Geometry: final body of the model. Coordinates: model frame, mm. A direction names the side the tool comes from. Coordinates: 2 decimals unless noted, no trailing zeros. Loops run counter-clockwise (first coordinate to the right, second up) from the corner with the lowest first, then second, coordinate; pieces in that order, holes last. Notation, with made-up numbers: (7, 15) - (14, 15) arc R25 cw to (14, 31) - close; hole circle Ø4 at (8, 62). An arc over 180 degrees is marked (long way). Answer in a Markdown table with one row per item.
from build123d import *

# Parameters (mm, degrees)
BOSS_EXTRUDE1_DEPTH   = 25.4
F_6_32_TAPPED_HOLE1_D = 2.7051
F_6_32_TAPPED_HOLE2_D = 2.7051
SKETCH7_R             = 1.5875
CUT_EXTRUDE1_DEPTH    = 4.048


with BuildPart() as part:
    # Sketch1 → Boss-Extrude1 (new body)
    with BuildSketch(Plane.XY):
        Polygon((0, 0), (19.05, 0), (19.05, 3.048), (3.048, 3.048), (3.048, 19.05), (0, 19.05), align=None)
    extrude(amount=BOSS_EXTRUDE1_DEPTH)

    # #6-32 Tapped Hole1 (through all)
    with Locations(Plane(origin=(3.048, 0, 0), x_dir=(0, 0, -1), z_dir=(1, 0, 0))):
        with Locations((-20.32, 9.525), (-5.08, 9.525)):
            Hole(F_6_32_TAPPED_HOLE1_D / 2)

    # #6-32 Tapped Hole2 (through all)
    with Locations(Plane(origin=(0, 3.048, 0), x_dir=(1, 0, 0), z_dir=(0, 1, 0))):
        with Locations((6, -20.65), (6, -4.65)):
            Hole(F_6_32_TAPPED_HOLE2_D / 2)

    # Sketch7 → Cut-Extrude1 (cut, through all)
    with BuildSketch(Plane(origin=(3.048, 0, 0), x_dir=(0, 0, -1), z_dir=(1, 0, 0))):
        with Locations((-20.32, 14.605)):
            Circle(SKETCH7_R)
        with Locations((-5.08, 14.605)):
            Circle(SKETCH7_R)
    extrude(amount=-CUT_EXTRUDE1_DEPTH, mode=Mode.SUBTRACT)


solid = part.part
(1) Cut plane C-C on z = 4.65. Output: boundary loops of the cut face in (x, y), then the cut area to 3 significant figures.
Verdict:
| item | result |
|---|---|
| outline | (0, 0) - (4.65, 0) - (4.65, 3.05) - (3.05, 3.05) - (3.05, 8.24) - (0, 8.24) - close; (0, 10.81) - (3.05, 10.81) - (3.05, 13.08) - (0, 13.08) - close; (0, 16.13) - (3.05, 16.13) - (3.05, 19.05) - (0, 19.05) - close; (7.35, 0) - (19.05, 0) - (19.05, 3.05) - (7.35, 3.05) - close |
| area | 81.5 mm² |
(2) First-contact query: pin 1 Ø8 at (y, z) = (10.5, 6.5) entering from +X; pin 2 Ø1.9 at (y, z) = (14.605, 5.08) entering from +X; pin 3 Ø5 at (x, z) = (7.5, 5.5) entering from +Y; pin 4 Ø8 at (y, z) = (3.5, 16.5) entering from +X. Flat tips, straight axial feed; report the tip coordinate or a pass-through.
Verdict:
| item | result |
|---|---|
| pin 1 | stops at x = 3.05 |
| pin 2 | passes through |
| pin 3 | stops at y = 3.05 |
| pin 4 | stops at x = 19.05 |
(3) Pull-direction query (X, two-part tool) for faces 3 (the face through (3.048, 11, 13)), 4 (the face through (5.38, 1.5, 21.85)), 5 (the face through (9, 0, 13)); classes: pulls with the +X half, pulls with the -X half, needs draft (parallel to the pull), parting line crosses it, or undercut.
Verdict:
| item | result |
|---|---|
| face 3 | pulls with the +X half |
| face 4 | undercut |
| face 5 | needs draft |
(4) Cut plane B-B on y = 8.5. Output: boundary loops of the cut face in (x, z).
Verdict:
| item | result |
|---|---|
| outline | (0, 0) - (3.05, 0) - (3.05, 4.2) - (0, 4.2) - close; (0, 5.96) - (3.05, 5.96) - (3.05, 19.44) - (0, 19.44) - close; (0, 21.2) - (3.05, 21.2) - (3.05, 25.4) - (0, 25.4) - close |
(5) Cut plane A-A on x = 6. Output: boundary loops of the cut face in (y, z), then the cut area to 3 significant figures.
Verdict:
| item | result |
|---|---|
| outline | (0, 0) - (3.05, 0) - (3.05, 3.3) - (0, 3.3) - close; (0, 6) - (3.05, 6) - (3.05, 19.3) - (0, 19.3) - close; (0, 22) - (3.05, 22) - (3.05, 25.4) - (0, 25.4) - close |
| area | 60.9 mm² |
(6) Cut plane D-D on z = 14. Output: boundary loops of the cut face in (x, y), then the cut area to 3 significant figures.
Verdict:
| item | result |
|---|---|
| outline | (0, 0) - (19.05, 0) - (19.05, 3.05) - (3.05, 3.05) - (3.05, 19.05) - (0, 19.05) - close |
| area | 107 mm² |
(7) Ray query, probe 1 along Z at (x, y) = (6, 1.25); probe 2 along Y at (x, z) = (0.75, 20.32); probe 3 along Z at (x, y) = (3, 16). Return the intervals inside material, ascending.
Verdict:
| item | result |
|---|---|
| probe 1 | z = 0 to 3.3, 6 to 19.3, 22 to 25.4 |
| probe 2 | y = 0 to 8.17, 10.88 to 13.02, 16.19 to 19.05 |
| probe 3 | z = 0 to 4.32, 5.84 to 19.56, 21.08 to 25.4 |
(8) Access query for faces 1 (the face through (11, 3.048, 13)), 2 (the face through (2, 6, 25.4)). Directions: +Z, -Z, +X, -X, +Y, -Y. A direction counts if a zero-diameter tool reaches every point of the face in a straight line with its end or side. Return the directions, or none.
Verdict:
| item | result |
|---|---|
| face 1 | +Z, -Z, +X, +Y |
| face 2 | +Z, +X, -X, +Y, -Y |
